from build123d import *

# Parameters (mm, degrees)
SKETCH1_W               = 100
SKETCH1_H               = 10
BOSS_EXTRUDE1_DEPTH     = 50
SKETCH2_W               = 5.031669049
SKETCH2_H               = 7.399484506
CUT_EXTRUDE1_DEPTH      = 112.915146428
MIRROR2_COPY_1_SKETCH_W = 5.031669049
MIRROR2_COPY_1_SKETCH_H = 7.399484506
MIRROR2_COPY_1_DEPTH    = 112.915146428
CUT_EXTRUDE2_DEPTH      = 72.414284285


with BuildPart() as part:
    # Sketch1 → Boss-Extrude1 (new, symmetric)
    with BuildSketch(Plane.XY):
        Rectangle(SKETCH1_W, SKETCH1_H)
    extrude(amount=BOSS_EXTRUDE1_DEPTH, both=True)

    # Sketch2 → Cut-Extrude1 (cut, through all)
    with BuildSketch(Plane.XY.offset(50)):
        with Locations((45.494674326, 0)):
            Rectangle(SKETCH2_W, SKETCH2_H)
    cut_extrude1 = extrude(amount=-CUT_EXTRUDE1_DEPTH, mode=Mode.SUBTRACT)

    # Mirror1: Cut-Extrude1 across plane
    add(cut_extrude1.mirror(Plane(origin=(0, 0, 0), x_dir=(0.7071067811865476, 0, 0.7071067811865476), z_dir=(-0.7071067811865477, 0, 0.7071067811865475))), mode=Mode.SUBTRACT)

    # Mirror2: Cut-Extrude1 across plane
    add(cut_extrude1.mirror(Plane(origin=(0, 0, 0), x_dir=(-0.7071067811865476, 0, 0.7071067811865476), z_dir=(-0.7071067811865477, 0, -0.7071067811865475))), mode=Mode.SUBTRACT)

    # Mirror2 copy 1 sketch → Mirror2 copy 1 (cut, through all)
    with BuildSketch(Plane(origin=(0, 0, -50), x_dir=(-1, 0, 0), z_dir=(0, 0, -1))):
        with Locations((45.494674326, 0)):
            Rectangle(MIRROR2_COPY_1_SKETCH_W, MIRROR2_COPY_1_SKETCH_H)
    extrude(amount=-MIRROR2_COPY_1_DEPTH, mode=Mode.SUBTRACT)

    # Sketch3 → Cut-Extrude2 (cut, through all)
    with BuildSketch(Plane(origin=(0, 5, 0), x_dir=(1, 0, 0), z_dir=(0, 1, 0))):
        Polygon((-226.207235665, -201.784596614), (-53.944301898, 27.606350902), (-24.696492293, 66.553689202), (147.566441474, 295.944636718), (-311.215453559, 640.470504252), (-684.989130698, 142.74127092), align=None)
    extrude(amount=-CUT_EXTRUDE2_DEPTH, mode=Mode.SUBTRACT)


solid = part.part
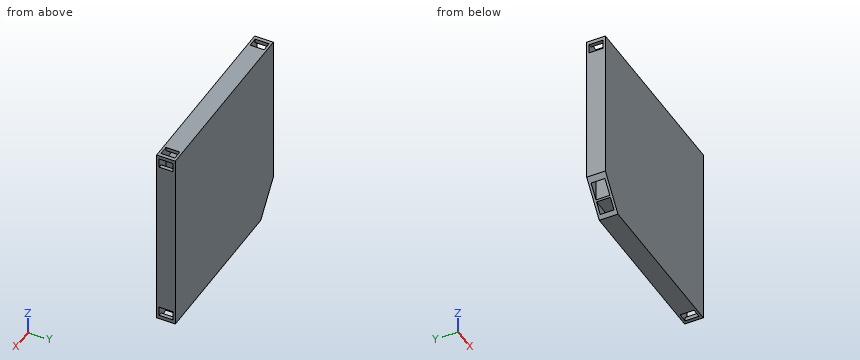
Verification items for the finished model (mm, model axes). Give positions to 0.01 mm unless a question says otherwise; leave off trailing zeros. Write each loop counter-clockwise with the first axis right and the second up, starting at its lowest first coordinate (ties: lowest second). Pieces come first, ordered by that corner, then holes. Notation, with made-up numbers: M -38.5,-5 L -30.5,-5 A16 cw -30.5,4 Z; hole C 70.5,62.5 d10. An arc over 180 degrees is marked long. Put each result on its own line as item: value. Start each with the question number.
1. Section check A-A (z = -15). Record the cut outline in (x, y).
2. Section check D-D (z = -40.5). Record the cut outline in (x, y), and give its area (3 significant figures).
3. Section check B-B (y = -1.5). Give the number of separate pieces and of enclosed holes in the cut face, and give its area (3 significant figures).
4. Section check C-C (x = -4.5). Record the cut outline in (y, z).
5. Scan lines: line 1 along X through (y, z) = (1, 40); line 2 along Y through (x, z) = (-45, -11.5). Record each from-to range of solid material in increasing order. Write a range as [from, to].
Answer list:
1. outline: M -50,-5 L 50,-5 L 50,5 L -50,5 Z; hole M -48.01,-3.7 L -42.98,-3.7 L -42.98,3.7 L -48.01,3.7 Z; hole M 42.98,-3.7 L 48.01,-3.7 L 48.01,3.7 L 42.98,3.7 Z
2. outline: M -44.26,-5 L 50,-5 L 50,5 L -44.26,5 L -44.26,3.7 L -42.98,3.7 L -42.98,-3.7 L -44.26,-3.7 Z; hole M 42.98,-3.7 L 48.01,-3.7 L 48.01,3.7 L 42.98,3.7 Z
2. area: 896 mm2
3. separate pieces: 8
3. enclosed holes: 0
3. area: 8,060 mm2
4. outline: M -5,-50 L 5,-50 L 5,50 L -5,50 Z; hole M -3.7,-48.01 L 3.7,-48.01 L 3.7,-42.98 L -3.7,-42.98 Z; hole M -3.7,42.98 L 3.7,42.98 L 3.7,48.01 L -3.7,48.01 Z
5. line 1: [-50, -48.01], [-42.98, 42.98], [48.01, 50]
5. line 2: [-5, -3.7], [3.7, 5]
